Build history of the part. All positions in model axes, mm. Face numbers are marked on the shaded views. A direction names the side the tool comes from. Round coordinates to 2 decimals unless told otherwise and drop trailing zeros. Write each loop counter-clockwise with the first axis right and the second up, starting at its lowest first coordinate (ties: lowest second). Pieces come first, ordered by that corner, then holes. Notation, with made-up numbers: M 65,75.5 L 121,75.5 A21 cw 121,85.5 Z; hole C 25,-38 d2. An arc over 180 degrees is marked long. Write item = value, one per line. Start each with the question number.
Q1. Probe L1, parallel to Z at x = 12, y = 7; L2, parallel to Y at x = -6, z = 5.25; L3, parallel to Y at x = 8.5, z = 1.75. List the from-to ranges inside material, lowest first.
Q2. Band-saw the part on B-B on z = 10.5. Write the cut outline in (x, y) (3 decimals).
Q3. Band-saw the part on C-C on y = -6.75. Write the cut outline in (x, z), plus the area to 3 significant figures.
Q4. Pull direction Y, two halves, no side cores. Call the marked faces 1, 2, 3 and 4: released by +Y, released by -Y, zero draft, split by the parting line, or undercut.
Q5. Drop flat-ended pins along their axis: P1, Ø5.5, axis at x = -3, z = 8, coming from the +Y side (3 decimals); P2, Ø2, axis at x = -3, y = -3, coming from the +Z side; P3, Ø6.5, axis at x = -15, z = 10.5, coming from the +Y side. Give the stop position or say it passes through.
Q6. Tool access for the marked faces 5, 6, 7, 8 and 9: list every direction of +Z, -Z, +X, -X, +Y, -Y with a clear straight run to the whole face (end or side of a thin tool).
Q7. Band-saw the part on A-A on x = 0. Write the cut outline in (y, z), plus the area to 3 significant figures.
Q8. Band-saw the part on D-D on y = 1. Write the cut outline in (x, z).
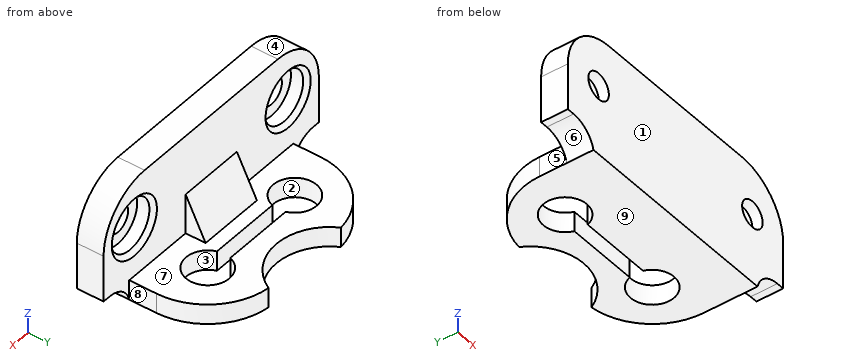
```python
from build123d import *

# Parameters (mm, degrees)
CROQUIS1_W                                  = 16.000027591
CROQUIS1_H                                  = 18
CROQUIS1_R                                  = 3.25
SALIENTE_EXTRUIR1_DEPTH                     = 3
CROQUIS2_W                                  = 15
CROQUIS2_H                                  = 2
CORTAR_EXTRUIR1_DEPTH                       = 3
REDONDEO1_R                                 = 10
CROQUIS3_W                                  = 15
CROQUIS3_H                                  = 4
SALIENTE_EXTRUIR2_DEPTH                     = 21
CROQUIS4_R                                  = 2
CORTAR_EXTRUIR2_DEPTH                       = 32
REDONDEO2_R                                 = 8
REFRENTADO_PARA_TORNILLO_CON_CABEZA_2_COUNT = 2
REFRENTADO_PARA_TORNILLO_CON_CABEZA_2_PITCH = 30
NERVIO1_REACH                               = 31.086
CROQUIS6_WALL_W                             = 66.880362222
CROQUIS6_WALL_H                             = 10
REDONDEO3_R                                 = 4


with BuildPart() as part:
    # Croquis1 → Saliente-Extruir1 (new body)
    # profile 1 of 2: a face of its own
    with BuildSketch(Plane.XY):
        with Locations((-8.000013796, 0)):
            Rectangle(CROQUIS1_W, CROQUIS1_H)
        with Locations((-8.5, 1)):
            Circle(CROQUIS1_R, mode=Mode.SUBTRACT)
    # profile 2 of 2: a face of its own
    with BuildSketch(Plane.XY):
        with Locations((8.000013796, 0)):
            Rectangle(CROQUIS1_W, CROQUIS1_H)
        with Locations((8.5, 1)):
            Circle(CROQUIS1_R, mode=Mode.SUBTRACT)
    extrude(amount=SALIENTE_EXTRUIR1_DEPTH)

    # Croquis2 → Cortar-Extruir1 (cut)
    with BuildSketch(Plane.XY.offset(3)):
        with BuildLine():
            ThreePointArc((7.068057866, 9), (7.76351927, 10.816597123), (8, 12.747340124))
            ThreePointArc((8, 12.747340124), (-1.930743001, 20.510859395), (-7.068057866, 9))
            Line((-7.068057866, 9), (7.068057866, 9))
        make_face()
        with BuildLine():
            Line((7.068057866, 9), (-7.068057866, 9))
            ThreePointArc((-7.068057866, 9), (0, 4.747340124), (7.068057866, 9))
        make_face()
        with Locations((0, 1)):
            Rectangle(CROQUIS2_W, CROQUIS2_H)
    extrude(amount=-CORTAR_EXTRUIR1_DEPTH, mode=Mode.SUBTRACT)

    # Redondeo1
    # the kernel refuses this fillet: 10 mm, written as the material it takes off along each edge
    with BuildSketch(Plane(origin=(16.000027591, 9, -24.857004965), x_dir=(-1, 0, 0), z_dir=(0, 0, 1))) as redondeo1_piece_1:
        with BuildLine():
            CenterArc((10, 9.942801986), REDONDEO1_R, 180, 83.86894335)
            Line((0, 9.942801986), (-0.2, 9.942801986))
            Line((-0.2, 9.942801986), (-0.2, 0))
            Line((-0.2, 0), (0, -0.2))
            ThreePointArc((0, -0.2), (4.465984863, -0.2), (8.91060912, -0.19885604))
            Line((8.91060912, -0.19885604), (8.931969726, 0))
        make_face()
    extrude(amount=52.71400993, mode=Mode.SUBTRACT)
    with BuildSketch(Plane(origin=(-16.000027591, 9, -24.857004965), x_dir=(1, 0, 0), z_dir=(0, 0, 1))) as redondeo1_piece_2:
        with BuildLine():
            CenterArc((10, -9.942801986), REDONDEO1_R, 96.13105665, 83.86894335)
            Line((0, -9.942801986), (-0.2, -9.942801986))
            Line((-0.2, -9.942801986), (-0.2, 0))
            Line((-0.2, 0), (0, 0.2))
            ThreePointArc((0, 0.2), (4.465984863, 0.2), (8.91060912, 0.19885604))
            Line((8.91060912, 0.19885604), (8.931969726, 0))
        make_face()
    extrude(amount=52.71400993, mode=Mode.SUBTRACT)

    # Croquis3 → Saliente-Extruir2 (add, symmetric)
    with BuildSketch(Plane(origin=(0, 0, 0), x_dir=(0, 0, -1), z_dir=(1, 0, 0))):
        with Locations((-10.5, -7)):
            Rectangle(CROQUIS3_W, CROQUIS3_H)
    extrude(amount=SALIENTE_EXTRUIR2_DEPTH, both=True)

    # Croquis4 → Cortar-Extruir2 (cut)
    with BuildSketch(Plane(origin=(0, -5, 0), x_dir=(1, 0, 0), z_dir=(0, 1, 0))):
        with Locations(Location((-15, -10.5, 0), (0, 0, 270))):
            Circle(CROQUIS4_R)
        with Locations(Location((15, -10.5, 0), (0, 0, 90))):
            Circle(CROQUIS4_R)
    extrude(amount=-CORTAR_EXTRUIR2_DEPTH, mode=Mode.SUBTRACT)

    # Redondeo2
    redondeo2_edges = [part.edges().sort_by_distance(p)[0] for p in [
        (-21, -7, 18),
        (21, -7, 18),
    ]]
    fillet(redondeo2_edges, radius=REDONDEO2_R)

    # Croquis5 → Refrentado para tornillo con cabeza troncocónica de #61 (revolve, cut)
    with BuildSketch(Plane(origin=(-15, -5, 10.5), x_dir=(0, 0, 1), z_dir=(1, 0, 0))):
        Polygon((0, 0), (0, 4), (1.89865, 4), (1.89865, 2.4638), (3.77063, 2.4638), (3.77063, 0.635), (4.40563, 0), align=None)
    refrentado_para_tornillo_con_cabeza_tron = revolve(axis=Axis((-15, 1.35, 10.5), (0, -1, 0)), mode=Mode.SUBTRACT)

    # Refrentado para tornillo con cabeza  2: Refrentado para tornillo con cabeza troncocónica de #61 ×2
    with Locations(*[(i * REFRENTADO_PARA_TORNILLO_CON_CABEZA_2_PITCH, 0, 0) for i in range(1, REFRENTADO_PARA_TORNILLO_CON_CABEZA_2_COUNT)]):
        add(refrentado_para_tornillo_con_cabeza_tron, mode=Mode.SUBTRACT)

    # Croquis6 wall → Nervio1 (add, up to next)
    with BuildSketch(Plane(origin=(0, -3.5, 6), x_dir=(0, -0.4472135955, 0.894427191), z_dir=(0, -0.894427191, -0.4472135955)), mode=Mode.PRIVATE) as nervio1_sk1:
        Rectangle(CROQUIS6_WALL_W, CROQUIS6_WALL_H)
    nervio1_tool1 = extrude(nervio1_sk1.sketch, amount=NERVIO1_REACH, mode=Mode.PRIVATE) - part.part
    add(nervio1_tool1.solids().sort_by_distance((0, -3.5, 6))[0])

    # Redondeo3
    # the kernel refuses this fillet: 4 mm, written as the material it adds along each edge
    with BuildSketch(Plane(origin=(16.000027591, -9, 3), x_dir=(0, 0, -1), z_dir=(0, 1, 0))) as redondeo3_piece_1:
        with BuildLine():
            CenterArc((4, -3.872983346), REDONDEO3_R, 104.477512186, 75.522487814)
            Line((0, -3.872983346), (0, 0))
            Line((0, 0), (3, 0))
        make_face()
    extrude(amount=4)
    with BuildSketch(Plane(origin=(-16.000027591, -9, 3), x_dir=(-1, 0, 0), z_dir=(0, 1, 0))) as redondeo3_piece_2:
        with BuildLine():
            CenterArc((3.872983346, -4), REDONDEO3_R, 90, 75.522487814)
            Line((0, -3), (0, 0))
            Line((0, 0), (3.872983346, 0))
        make_face()
    extrude(amount=4)


solid = part.part
```
Conclusion:
q1.L1 = 0 to 3
q1.L2 = -9 to -5
q1.L3 = -9 to -2.25, 4.25 to 8.74
q2.outline = M -20.984,-9 L -17,-9 L -17,-7.464 L -18.771,-7.464 L -18.771,-5.635 L -19.406,-5 L -20.984,-5 Z; M -13,-9 L 13,-9 L 13,-7.464 L 11.229,-7.464 L 11.229,-5.635 L 10.594,-5 L -10.594,-5 L -11.229,-5.635 L -11.229,-7.464 L -13,-7.464 Z; M 17,-9 L 20.984,-9 L 20.984,-5 L 19.406,-5 L 18.771,-5.635 L 18.771,-7.464 L 17,-7.464 Z
q3.outline = M -21,3 L -19.87,3 A4 cw -16,0 L 16,0 A4 cw 19.87,3 L 21,3 L 21,10 A8 ccw 13,18 L -13,18 A8 ccw -21,10 Z; hole C -15,10.5 d7.54; hole C 15,10.5 d7.54
q3.area = 615 mm^2
q4.face_1 = released by -Y
q4.face_2 = undercut
q4.face_3 = undercut
q4.face_4 = zero draft
q5.P1 = -3.125
q5.P2 = 7
q5.P3 = -7.46
q6.face_5 = +Z, -Z, -X, +Y
q6.face_6 = -Z, -X, +Y, -Y
q6.face_7 = +Z, +Y
q6.face_8 = +Z, -Z, +X, +Y
q6.face_9 = -Z, +X, -X, +Y, -Y
q7.outline = M -9,0 L 0,0 L 0,3 L -2,3 L -5,9 L -5,18 L -9,18 Z; M 2,0 L 4.75,0 L 4.75,3 L 2,3 Z
q7.area = 104 mm^2
q8.outline = M -15.81,0 L -11.75,0 L -11.75,3 L -15.81,3 Z; M 11.75,0 L 15.81,0 L 15.81,3 L 11.75,3 Z
